The listing builds one solid part. Answer for the finished solid, in the listing's coordinates (mm). Coordinates: 2 decimals unless noted, no trailing zeros. Write each loop counter-clockwise with the first axis right and the second up, starting at its lowest first coordinate (ties: lowest second). Pieces come first, ordered by that corner, then holes. Notation, with made-up numbers: M 78.25,76 L 93.25,76 A11 cw 93.25,90 Z; hole C 49.5,80 d9. An arc over 180 degrees is marked long. Answer as CSV lines item,"result".
```python
from build123d import *

# Parameters (mm, degrees)
F0_R     = 2.794
F1_DEPTH = 139.7
F2_R     = 6.35
F3_DEPTH = 9.525
F4_R     = 1.27
F5_R     = 0.254
F6_R     = 2.460798
F7_DEPTH = 25.4
F8_DEPTH = 25.4


with BuildPart() as f1:
    # F0 (on Top) → F1 (new body)
    with BuildSketch(Plane.XY):
        Circle(F0_R)
    extrude(amount=F1_DEPTH)

    # F2 (on face) → F3 (join)
    with BuildSketch(Plane(origin=(0, 0, 0), x_dir=(1, 0, 0), z_dir=(0, 0, -1))):
        Circle(F2_R)
    extrude(amount=-F3_DEPTH)

    # F4
    f4_edges = [f1.edges().sort_by_distance(p)[0] for p in [
        (-2.794, 0, 9.525),
    ]]
    fillet(f4_edges, radius=F4_R)

    # F5
    f5_edges = [f1.edges().sort_by_distance(p)[0] for p in [
        (-6.35, 0, 9.525),
    ]]
    fillet(f5_edges, radius=F5_R)

    # F6 (on Right) → F7 (cut)
    with BuildSketch(Plane.YZ):
        with Locations((0, 4.7625)):
            Circle(F6_R)
    extrude(amount=-F7_DEPTH, mode=Mode.SUBTRACT)

    # F6 (on Right) → F8 (cut)
    with BuildSketch(Plane.YZ):
        with Locations((0, 4.7625)):
            Circle(F6_R)
    extrude(amount=F8_DEPTH, mode=Mode.SUBTRACT)


solid = f1.part
```
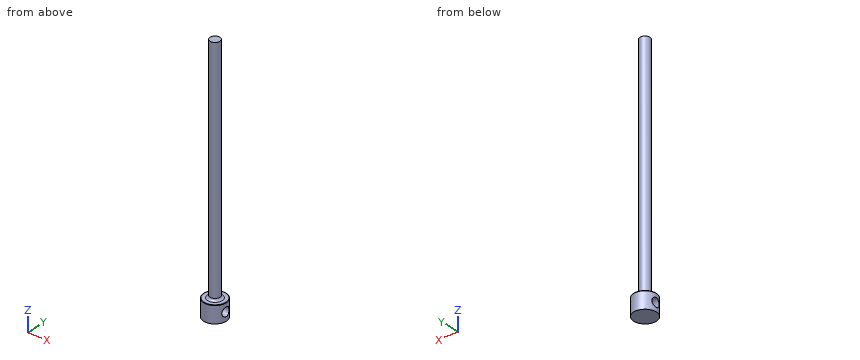
Q1. Straight lines are drawn through the part: line 1 (Z direction, x = 5, y = 0) (3 decimals); line 2 (Z direction, x = -1.5, y = 0); line 3 (Z direction, x = 3, y = -4) (3 decimals). For each, find the intervals that lie inside material, in ascending order.
Output:
line 1,"0 to 2.302, 7.223 to 9.525"
line 2,"0 to 2.3, 7.22 to 139.7"
line 3,"0 to 9.525"
Q2. Find section A-A (y = 0). Give the vertices of the cut face in (x, z) (3 decimals).
Output:
outline,"M -6.35,0 L 6.35,0 L 6.35,2.302 L -6.35,2.302 Z; M -6.35,7.223 L 6.35,7.223 L 6.35,9.271 A0.254 ccw 6.096,9.525 L 4.064,9.525 A1.27 cw 2.794,10.795 L 2.794,139.7 L -2.794,139.7 L -2.794,10.795 A1.27 cw -4.064,9.525 L -6.096,9.525 A0.254 ccw -6.35,9.271 Z"
Q3. Flat-ended cylindrical pins translate along their axes: pin 1 Ø6 at (x, y) = (0, 4.5) entering from +Z; pin 2 Ø5 at (y, z) = (-0.5, 59.5) entering from -X; pin 3 Ø4 at (y, z) = (0, 26) entering from +X; pin 4 Ø5 at (x, z) = (3, 120.5) entering from +Y. Find the tip coordinate at first contact, or state that the pin passes through.
Output:
pin 1,"z = 139.7"
pin 2,"x = -2.79"
pin 3,"x = 2.79"
pin 4,"y = 2.75"
Q4. Find section B-B (z = 101.5). Give the vertices of the cut face in (x, y), and give its area (3 significant figures).
Output:
outline,"C 0,0 d5.59"
area,"24.5 mm2"
